The listing builds one solid part. Answer for the finished solid, in the listing's coordinates (mm). A direction names the side the tool comes from. Give positions to 0.01 mm unless a question says otherwise; leave off trailing zeros. Loops run counter-clockwise (first coordinate to the right, second up) from the corner with the lowest first, then second, coordinate; pieces in that order, holes last.
Item 1: Section A-A, the plane y = 0 is taken. Give the vertices of the cut face in (x, z), and give its area (3 significant figures).
Item 2: Consider line 1 along X through (y, z) = (0, 2.75); line 2 along Y through (x, z) = (0, 6.5); line 3 along Z through (x, y) = (48.5, 25). Determine where each line is inside the solid, lowest interval first.
Item 3: The mould has two halves that part along Y. Classify faces 1 (the face through (43.876, 13.817, 4.93)), 2 (the face through (26.34, 41.32, 5.46)), 3 (the face through (41, 41, 2)), 4 (the face through (-28, 41, 0)): pulls with the +Y half, pulls with the -Y half, needs draft (parallel to the pull), parting line crosses it, or undercut.
Item 4: A tool of negligible diameter and unlimited length cuts with its end or side. For faces 5 (the face through (-28, 41, 3)), 6 (the face through (60, -1, 1)), 7 (the face through (-41, 41, 2)), from which of +Z, -Z, +X, -X, +Y, -Y can it reach the whole face along a straight path? Write none if from no direction.
Item 5: Each of these flat-tipped pins is pushed along its axis until it touches: pin 1 Ø1.5 at (y, z) = (38.5, 5.5) entering from -X; pin 2 Ø2 at (x, z) = (7.5, 8) entering from -Y; pin 3 Ø6 at (x, y) = (40.5, -39.5) entering from -Z. Where does it stop, or does it pass through?
from build123d import *

# Parameters (mm, degrees)
F0_R     = 49
F0_R_2   = 46
F1_DEPTH = 10
F0_W     = 120
F0_H     = 120
F2_DEPTH = 3
F3_SIZE  = 2
F5_DEPTH = 2
F6_R     = 5


with BuildPart() as f1:
    # F0 (on Top) → F1 (new body)
    with BuildSketch(Plane.XY):
        Circle(F0_R)
        Circle(F0_R_2, mode=Mode.SUBTRACT)
    extrude(amount=F1_DEPTH)

    # F0 (on Top) → F2 (join)
    with BuildSketch(Plane.XY):
        Rectangle(F0_W, F0_H)
        Circle(F0_R, mode=Mode.SUBTRACT)
    extrude(amount=F2_DEPTH)

    # F3
    f3_edges = [f1.edges().sort_by_distance(p)[0] for p in [
        (-49, 0, 10),
    ]]
    chamfer(f3_edges, length=F3_SIZE)

    # F4 (on face) → F5 (cut)
    with BuildSketch(Plane(origin=(0, 0, 0), x_dir=(1, 0, 0), z_dir=(0, 0, -1))):
        Polygon((-27.604349, 36.796738), (-41.746485, 50.938873), (-50.938873, 41.746485), (-36.796738, 27.604349), align=None)
        Polygon((41.746485, -50.938873), (50.938873, -41.746485), (36.796738, -27.604349), (27.604349, -36.796738), align=None)
        Polygon((50.938873, 41.746485), (41.746485, 50.938873), (27.604349, 36.796738), (36.796738, 27.604349), align=None)
        Polygon((-36.796738, -27.604349), (-50.938873, -41.746485), (-41.746485, -50.938873), (-27.604349, -36.796738), align=None)
    extrude(amount=-F5_DEPTH, mode=Mode.SUBTRACT)

    # F6
    f6_edges = [f1.edges().sort_by_distance(p)[0] for p in [
        (-32.526912, -32.526912, 2),
        (32.526912, -32.526912, 2),
        (32.526912, 32.526912, 2),
        (-32.526912, 32.526912, 2),
    ]]
    fillet(f6_edges, radius=F6_R)


solid = f1.part
Worked answers:
1. outline: (-60, 0) - (-46, 0) - (-46, 10) - (-47, 10) - (-49, 8) - (-49, 3) - (-60, 3) - close; (46, 0) - (60, 0) - (60, 3) - (49, 3) - (49, 8) - (47, 10) - (46, 10) - close
1. area: 122 mm2
2. line 1: x = -60 to -46, 46 to 60
2. line 2: y = -49 to -46, 46 to 49
2. line 3: z = 0 to 3
3. face 1: undercut
3. face 2: parting line crosses it
3. face 3: undercut
3. face 4: needs draft
4. face 5: +Z
4. face 6: +Z, -Z, +X, +Y, -Y
4. face 7: -Z
5. pin 1: stops at x = -31.24
5. pin 2: stops at y = -48.57
5. pin 3: stops at z = 2
